Can you work these out from the model? Positions are in its coordinate system, mm. A direction names the side the tool comes from. Give positions to 0.01 mm unless a question says otherwise; leave off trailing zeros. Order: outer loops, then holes, each group sorted by start corner. A loop starts at its lowest first (then second) coordinate and runs counter-clockwise, first axis right, second up. Notation, with made-up numbers: (-18.5, -33.5) -> (8.5, -33.5) arc R23 cw to (8.5, -9.5) -> close; hole circle Ø11 at (18.5, 88.25). An arc over 180 degrees is marked (long way). Answer as CSV lines item,"result".
```python
from build123d import *

# Parameters (mm, degrees)
BOSS_EXTRUDE1_DEPTH      = 35
BOSS_EXTRUDE2_DEPTH      = 35
FILLET1_R                = 0.5
SKETCH3_W                = 26
SKETCH3_H                = 25
CUT_EXTRUDE1_DEPTH       = 1.5
SKETCH4_W                = 16
SKETCH4_H                = 25
CUT_EXTRUDE2_DEPTH       = 2
FILLET3_R                = 1
SKETCH5_W                = 26
SKETCH5_H                = 25
CUT_EXTRUDE3_DEPTH       = 1.5
SKETCH6_W                = 16
SKETCH6_H                = 25
CUT_EXTRUDE4_DEPTH       = 2
FILLET4_R                = 1
SKETCH8_W                = 20
SKETCH8_H                = 3
CUT_EXTRUDE5_DEPTH       = 4
SKETCH9_W                = 20
SKETCH9_H                = 3
CUT_EXTRUDE6_DEPTH       = 4
SKETCH10_W               = 20
SKETCH10_H               = 3
CUT_EXTRUDE7_DEPTH       = 4
SKETCH11_R               = 1.1
CUT_EXTRUDE8_DEPTH       = 10
SKETCH12_R               = 1.1
CUT_EXTRUDE9_DEPTH       = 5
FILLET7_R                = 2
BOSS_EXTRUDE3_DEPTH      = 3.5
BOSS_EXTRUDE3_DEPTH_BACK = 1
SKETCH14_W               = 35
SKETCH14_H               = 3.801557548
SKETCH15_W               = 1.5
SKETCH15_H               = 31
CUT_EXTRUDE10_DEPTH      = 5
SKETCH18_R               = 1.1
SKETCH18_W               = 16
SKETCH18_H               = 20
BOSS_EXTRUDE4_DEPTH      = 6.5
SKETCH19_R               = 1.1
SKETCH19_W               = 16
SKETCH19_H               = 17.5
BOSS_EXTRUDE5_DEPTH      = 6.5


with BuildPart() as part:
    # Sketch1 → Boss-Extrude1 (new body)
    with BuildSketch(Plane.XY):
        Polygon((6.55, 4.55), (-6.55, 4.55), (-6.55, -4.55), (-2.05, -4.55), (-2.05, -2.05), (-4.05, -2.05), (-4.05, 2.05), (4.05, 2.05), (4.05, -2.05), (2.05, -2.05), (2.05, -4.55), (6.55, -4.55), align=None)
    extrude(amount=BOSS_EXTRUDE1_DEPTH)

    # Sketch2 → Boss-Extrude2 (add, through all)
    with BuildSketch(Plane.XY.offset(35)):
        Polygon((2, 4.55), (2, 25.472649731), (39.72114317, 47.250961894), (38.22114317, 49.849038106), (0.618900538, 28.1393732), (-19.093062702, 66.826279338), (-21.766082275, 65.464307839), (-2, 26.671187114), (-2, 4.55), align=None)
    extrude(amount=-BOSS_EXTRUDE2_DEPTH)

    # Fillet1
    fillet1_edges = [part.edges().sort_by_distance(p)[0] for p in [
        (0.618900538, 28.1393732, 17.5),
    ]]
    fillet(fillet1_edges, radius=FILLET1_R)

    # Sketch3 → Cut-Extrude1 (cut)
    with BuildSketch(Plane(origin=(-12.029980884, 20.836538106, 0), x_dir=(0, 0, 1), z_dir=(-0.4999999999999978, 0.8660254037844398, 0))):
        with Locations((17.5, 42.525)):
            Rectangle(SKETCH3_W, SKETCH3_H)
    extrude(amount=-CUT_EXTRUDE1_DEPTH, mode=Mode.SUBTRACT)

    # Sketch4 → Cut-Extrude2 (cut)
    with BuildSketch(Plane(origin=(-11.279980884, 19.5375, 0), x_dir=(0, 0, 1), z_dir=(-0.49999999999999795, 0.8660254037844399, 0))):
        with Locations((17.5, 42.525)):
            Rectangle(SKETCH4_W, SKETCH4_H)
    extrude(amount=-CUT_EXTRUDE2_DEPTH, mode=Mode.SUBTRACT)

    # Fillet3
    fillet3_edges = [part.edges().sort_by_distance(p)[0] for p in [
        (36.748066959, 46.400480947, 9.5),
        (36.748066959, 46.400480947, 25.5),
        (15.097431864, 33.900480947, 25.5),
        (15.097431864, 33.900480947, 9.5),
    ]]
    fillet(fillet3_edges, radius=FILLET3_R)

    # Sketch5 → Cut-Extrude3 (cut)
    with BuildSketch(Plane(origin=(11.873956138, 6.050082838, 0), x_dir=(0, 0, -1), z_dir=(0.8910065241883675, 0.45399049973954786, 0))):
        with Locations((-17.5, 52.710719955)):
            Rectangle(SKETCH5_W, SKETCH5_H)
    extrude(amount=-CUT_EXTRUDE3_DEPTH, mode=Mode.SUBTRACT)

    # Sketch6 → Cut-Extrude4 (cut)
    with BuildSketch(Plane(origin=(10.537446352, 5.369097089, 0), x_dir=(0, 0, -1), z_dir=(0.8910065241883673, 0.4539904997395479, 0))):
        with Locations((-17.5, 52.710719955)):
            Rectangle(SKETCH6_W, SKETCH6_H)
    extrude(amount=-CUT_EXTRUDE4_DEPTH, mode=Mode.SUBTRACT)

    # Fillet4
    fillet4_edges = [part.edges().sort_by_distance(p)[0] for p in [
        (-19.735855882, 63.131781141, 25.5),
        (-19.735855882, 63.131781141, 9.5),
        (-8.386093389, 40.856618036, 9.5),
        (-8.386093389, 40.856618036, 25.5),
    ]]
    fillet(fillet4_edges, radius=FILLET4_R)

    # Sketch8 → Cut-Extrude5 (cut)
    with BuildSketch(Plane(origin=(-10.529980884, 18.238461894, 0), x_dir=(0, 0, -1), z_dir=(0.49999999999999806, -0.8660254037844399, 0))):
        with Locations((-17.5, 24.025)):
            Rectangle(SKETCH8_W, SKETCH8_H)
    extrude(amount=-CUT_EXTRUDE5_DEPTH, mode=Mode.SUBTRACT)

    # Sketch9 → Cut-Extrude6 (cut)
    with BuildSketch(Plane(origin=(9.200936565, 4.688111339, 0), x_dir=(0, 0, 1), z_dir=(-0.8910065241883675, -0.45399049973954797, 0))):
        with Locations((17.5, 34.210719955)):
            Rectangle(SKETCH9_W, SKETCH9_H)
    extrude(amount=-CUT_EXTRUDE6_DEPTH, mode=Mode.SUBTRACT)

    # Sketch10 → Cut-Extrude7 (cut)
    with BuildSketch(Plane.ZY.offset(2)):
        with Locations((17.5, 15.062177826)):
            Rectangle(SKETCH10_W, SKETCH10_H)
    extrude(amount=-CUT_EXTRUDE7_DEPTH, mode=Mode.SUBTRACT)

    # Sketch11 → Cut-Extrude8 (cut)
    with BuildSketch(Plane(origin=(-11.279980884, 19.5375, 0), x_dir=(0, 0, 1), z_dir=(-0.4999999999999979, 0.8660254037844398, 0))):
        with Locations(Location((28, 52.525, 0), (0, 0, 270))):
            Circle(SKETCH11_R)
        with Locations(Location((7, 52.525, 0), (0, 0, 270))):
            Circle(SKETCH11_R)
        with Locations(Location((28, 40.025, 0), (0, 0, 270))):
            Circle(SKETCH11_R)
        with Locations(Location((7, 40.025, 0), (0, 0, 270))):
            Circle(SKETCH11_R)
    extrude(amount=-CUT_EXTRUDE8_DEPTH, mode=Mode.SUBTRACT)

    # Sketch12 → Cut-Extrude9 (cut)
    with BuildSketch(Plane(origin=(10.537446352, 5.369097089, 0), x_dir=(0, 0, -1), z_dir=(0.8910065241883673, 0.4539904997395479, 0))):
        with Locations(Location((-7, 62.710719955, 0), (0, 0, 90))):
            Circle(SKETCH12_R)
        with Locations(Location((-28, 62.710719955, 0), (0, 0, 90))):
            Circle(SKETCH12_R)
        with Locations(Location((-7, 50.210719955, 0), (0, 0, 90))):
            Circle(SKETCH12_R)
        with Locations(Location((-28, 50.210719955, 0), (0, 0, 90))):
            Circle(SKETCH12_R)
    extrude(amount=-CUT_EXTRUDE9_DEPTH, mode=Mode.SUBTRACT)

    # Fillet7
    fillet7_edges = [part.edges().sort_by_distance(p)[0] for p in [
        (-20.429572488, 66.145293588, 0),
        (38.97114317, 48.55, 0),
        (38.97114317, 48.55, 35),
        (-20.429572488, 66.145293588, 35),
    ]]
    fillet(fillet7_edges, radius=FILLET7_R)

    # Sketch14 → Boss-Extrude3 (add, two sides: drawn at the far end of the back side and taken through both)
    with BuildSketch(Plane(origin=(6.55, 0, 0), x_dir=(0, 0, -1), z_dir=(1, 0, 0)).offset(-BOSS_EXTRUDE3_DEPTH_BACK)):
        with Locations((-17.5, -0.05)):
            Rectangle(SKETCH14_W, SKETCH14_H)
    extrude(amount=BOSS_EXTRUDE3_DEPTH + BOSS_EXTRUDE3_DEPTH_BACK)

    # Sketch15 → Cut-Extrude10 (cut)
    with BuildSketch(Plane(origin=(0, 1.850778774, 0), x_dir=(1, 0, 0), z_dir=(0, 1, 0))):
        with Locations((7.3, -17.5)):
            Rectangle(SKETCH15_W, SKETCH15_H)
    extrude(amount=-CUT_EXTRUDE10_DEPTH, mode=Mode.SUBTRACT)

    # Sketch18 → Boss-Extrude4 (add)
    with BuildSketch(Plane(origin=(-10.529980884, 18.238461894, 0), x_dir=(0, 0, -1), z_dir=(0.49999999999999806, -0.8660254037844398, 0))):
        with BuildLine():
            Line((-35, 28.025), (-35, 56.025))
            ThreePointArc((-35, 56.025), (-34.414213562, 57.439213562), (-33, 58.025))
            Line((-33, 58.025), (-2, 58.025))
            ThreePointArc((-2, 58.025), (-0.585786438, 57.439213562), (0, 56.025))
            Line((0, 56.025), (0, 28.025))
            Line((0, 28.025), (-35, 28.025))
        make_face()
        with Locations(Location((-7, 52.525, 0), (0, 0, 270))):
            Circle(SKETCH18_R, mode=Mode.SUBTRACT)
        with Locations(Location((-7, 40.025, 0), (0, 0, 270))):
            Circle(SKETCH18_R, mode=Mode.SUBTRACT)
        with Locations(Location((-28, 40.025, 0), (0, 0, 270))):
            Circle(SKETCH18_R, mode=Mode.SUBTRACT)
        with Locations(Location((-28, 52.525, 0), (0, 0, 270))):
            Circle(SKETCH18_R, mode=Mode.SUBTRACT)
        with Locations((-17.5, 43.525)):
            Rectangle(SKETCH18_W, SKETCH18_H, mode=Mode.SUBTRACT)
    extrude(amount=BOSS_EXTRUDE4_DEPTH)

    # Sketch19 → Boss-Extrude5 (add)
    with BuildSketch(Plane(origin=(9.200936565, 4.688111339, 0), x_dir=(0, 0, 1), z_dir=(-0.8910065241883673, -0.45399049973954797, 0))):
        with BuildLine():
            Line((33, 68.210719955), (2, 68.210719955))
            ThreePointArc((2, 68.210719955), (0.585786438, 67.624933517), (0, 66.210719955))
            Line((0, 66.210719955), (0, 37.710719955))
            Line((0, 37.710719955), (35, 37.710719955))
            Line((35, 37.710719955), (35, 66.210719955))
            ThreePointArc((35, 66.210719955), (34.414213562, 67.624933517), (33, 68.210719955))
        make_face()
        with Locations(Location((28, 50.210719955, 0), (0, 0, 90))):
            Circle(SKETCH19_R, mode=Mode.SUBTRACT)
        with Locations(Location((7, 50.210719955, 0), (0, 0, 90))):
            Circle(SKETCH19_R, mode=Mode.SUBTRACT)
        with Locations(Location((7, 62.710719955, 0), (0, 0, 90))):
            Circle(SKETCH19_R, mode=Mode.SUBTRACT)
        with Locations(Location((28, 62.710719955, 0), (0, 0, 90))):
            Circle(SKETCH19_R, mode=Mode.SUBTRACT)
        with Locations((17.5, 51.960719955)):
            Rectangle(SKETCH19_W, SKETCH19_H, mode=Mode.SUBTRACT)
    extrude(amount=BOSS_EXTRUDE5_DEPTH)


solid = part.part
```
Item 1: Imagine slicing it at A-A, the plane z = 17.5. Give the number of separate pieces and of enclosed holes in the cut face, then the cut area to 3 significant figures.
Numbers:
separate pieces,"7"
enclosed holes,"0"
area,"404 mm²"
Item 2: Please list where these lines run through material, in increasing order: line 1 along X through (y, z) = (-1, 6); line 2 along Z through (x, y) = (-10, 48.5); line 3 along Z through (x, y) = (20.5, 33.5).
Numbers:
line 1,"x = -6.55 to -4.05, 4.05 to 6.55, 8.05 to 10.05"
line 2,"z = 0 to 4.5, 30.5 to 35"
line 3,"z = 0 to 9.5, 25.5 to 35"
Item 3: We'd pull the mould along X, two halves only. Please class faces 1 (the cylindrical face through (-16.04, 48.84, 6.07)), 2 (the cylindrical face through (35.3, 41.876, 7.421)), 3 (the flat face through (-4, 4.55, 17)), 4 (the flat face through (10.05, 0, 18)): released by +X, released by -X, zero draft, split by the parting line, or undercut.
Numbers:
face 1,"undercut"
face 2,"undercut"
face 3,"zero draft"
face 4,"released by +X"
Item 4: For faces 5 (the flat face through (4.05, 0, 17)), 6 (the flat face through (-19.397, 60.815, 17.388)), 7 (the flat face through (-17, 50, 9.5)), 8 (the flat face through (15.34, 29.48, 17.26)), which set-ups out of +Z, -Z, +X, -X, +Y, -Y let a thin tool reach every point of the face, with its end or its side?
Numbers:
face 5,"+Z, -Z"
face 6,"+X"
face 7,"none"
face 8,"+Z, -Z, -Y"
Item 5: For pin 1 (1.6 mm diameter, centred on x = -3.5, z = 18.5, fed in from +Y); pin 2 (1.9 mm diameter, centred on y = -0.5, z = 9, fed in from +X); pin 3 (6 mm diameter, centred on y = 35.5, z = 23, fed in from -X); pin 4 (3 mm diameter, centred on x = 8, z = 10.5, fed in from -Y), each with a flat end and sliding along its axis, tell me the tip position at first contact or that it passes through.
Numbers:
pin 1,"stops at y = 35.2"
pin 2,"stops at x = 10.05"
pin 3,"stops at x = -15.32"
pin 4,"stops at y = -4.55"
Item 6: Imagine slicing it at C-C, the plane y = 20. Please give me the cut outline in (x, z).
Numbers:
outline,"(-2, 0) -> (2, 0) -> (2, 35) -> (-2, 35) -> close"
